from build123d import *

# Parameters (mm, degrees)
BOSS_EXTRUDE1_DEPTH             = 7.6708
SKETCH2_W                       = 5.08
SKETCH2_H                       = 0.3048
CUT_EXTRUDE1_DEPTH              = 38.1
LPATTERN1_COUNT                 = 8
LPATTERN1_PITCH                 = 0.762
F_10_32_TAPPED_HOLE1_AT_2_COUNT = 2
F_10_32_TAPPED_HOLE1_AT_2_PITCH = 19.05


with BuildPart() as part:
    # Sketch1 → Boss-Extrude1 (new body)
    with BuildSketch(Plane.XY):
        with BuildLine():
            Line((52.1716, 20.6375), (54.409054124, 20.6375))
            ThreePointArc((54.409054124, 20.6375), (54.797860491, 20.560161605), (55.127474613, 20.33992049))
            Line((55.127474613, 20.33992049), (62.03402049, 13.433374613))
            ThreePointArc((62.03402049, 13.433374613), (62.254261605, 13.103760491), (62.3316, 12.714954124))
            Line((62.3316, 12.714954124), (62.3316, 6.335045876))
            ThreePointArc((62.3316, 6.335045876), (62.254261605, 5.946239509), (62.03402049, 5.616625387))
            Line((62.03402049, 5.616625387), (60.009497552, 3.592102448))
            ThreePointArc((60.009497552, 3.592102448), (58.5216, 0), (60.009497552, -3.592102448))
            Line((60.009497552, -3.592102448), (62.03402049, -5.616625387))
            ThreePointArc((62.03402049, -5.616625387), (62.254261605, -5.946239509), (62.3316, -6.335045876))
            Line((62.3316, -6.335045876), (62.3316, -12.714954124))
            ThreePointArc((62.3316, -12.714954124), (62.254261605, -13.103760491), (62.03402049, -13.433374613))
            Line((62.03402049, -13.433374613), (55.127474613, -20.33992049))
            ThreePointArc((55.127474613, -20.33992049), (54.797860491, -20.560161605), (54.409054124, -20.6375))
            Line((54.409054124, -20.6375), (52.1716, -20.6375))
            ThreePointArc((52.1716, -20.6375), (50.914364143, -20.116735857), (50.3936, -18.8595))
            Line((50.3936, -18.8595), (50.3936, 18.8595))
            ThreePointArc((50.3936, 18.8595), (50.914364143, 20.116735857), (52.1716, 20.6375))
        make_face()
    extrude(amount=-BOSS_EXTRUDE1_DEPTH)

    # Sketch2 → Cut-Extrude1 (cut, symmetric)
    with BuildSketch(Plane(origin=(0, 0, 0), x_dir=(1, 0, 0), z_dir=(0, 1, 0))):
        with Locations((49.4284, 0.9144)):
            Rectangle(SKETCH2_W, SKETCH2_H)
    cut_extrude1 = extrude(amount=CUT_EXTRUDE1_DEPTH, both=True, mode=Mode.SUBTRACT)

    # LPattern1: Cut-Extrude1 ×8
    with Locations(*[(0, 0, -i * LPATTERN1_PITCH) for i in range(1, LPATTERN1_COUNT)]):
        add(cut_extrude1, mode=Mode.SUBTRACT)

    # Sketch3 → #10-32 Tapped Hole1 (revolve, cut)
    with BuildSketch(Plane(origin=(56.3626, 9.525, 0), x_dir=(0, -1, 0), z_dir=(1, 0, 0))):
        Polygon((0, 0), (0, 7.6708), (2.54, 7.6708), (2.0193, 7.1501), (2.0193, 0.5207), (2.54, 0), align=None)
    f_10_32_tapped_hole1 = revolve(axis=Axis((56.3626, 9.525, 6.35), (0, 0, -1)), mode=Mode.SUBTRACT)

    # #10-32 Tapped Hole1 at 2: #10-32 Tapped Hole1 ×2
    with Locations(*[(0, -i * F_10_32_TAPPED_HOLE1_AT_2_PITCH, 0) for i in range(1, F_10_32_TAPPED_HOLE1_AT_2_COUNT)]):
        add(f_10_32_tapped_hole1, mode=Mode.SUBTRACT)


solid = part.part
Work out the finished part from the listing and answer in its coordinate system (mm). A direction names the side the tool comes from. Coordinates: 2 decimals unless noted, no trailing zeros. Write each loop counter-clockwise with the first axis right and the second up, starting at its lowest first coordinate (ties: lowest second). Pieces come first, ordered by that corner, then holes.
1. For faces 4 (the flat face through (51, 0, -5.639)), 5 (the flat face through (61.04, 4.62, -3.78)), 6 (the flat face through (55, 0, 0)), determine the directions among +Z, -Z, +X, -X, +Y, -Y from which every point of the face is accessible in a straight line to the end or side of a thin tool.
Results list:
face 4: -X, +Y, -Y
face 5: +Z, -Z, +X
face 6: +Z, +X, -X, +Y, -Y
2. Consider line 1 along Y through (x, z) = (55, -1); line 2 along Y through (x, z) = (57, -6.75); line 3 along X through (y, z) = (7, -1). Determine where each line is inside the solid, lowest interval first.
Results list:
line 1: y = -20.45 to -11.02, -8.03 to 8.03, 11.02 to 20.45
line 2: y = -18.47 to -11.44, -7.61 to 7.61, 11.44 to 18.47
line 3: x = 51.97 to 62.33
3. For a pull along X with two mould halves and no side action, classify faces 1 (the flat face through (55, 0, -7.671)), 2 (the flat face through (58.63, -16.84, -3.78)), 3 (the cylindrical face through (58.154, -10.457, -3.789)) as +X half, -X half, draft (parallel to the pull), parting line (faces both ways), or undercut.
Results list:
face 1: draft
face 2: +X half
face 3: undercut
4. The part is cut by section B-B, the plane x = 51.5. State how many separate pieces and enclosed holes the cut face has, and give its area (3 significant figures).
Results list:
separate pieces: 9
enclosed holes: 0
area: 215 mm2
5. The part is cut by section A-A, the plane x = 60.75. Write down the section's boundary in (y, z).
Results list:
outline: (-14.72, -7.67) - (-4.33, -7.67) - (-4.33, 0) - (-14.72, 0) - close; (4.33, -7.67) - (14.72, -7.67) - (14.72, 0) - (4.33, 0) - close
6. A flat-ended cylindrical pin translates along its axis: pin 1 (3 mm diameter, centred on y = 0, z = -2, fed in from +X). Find the tip coordinate at first contact, or state that the pin passes through.
Results list:
pin 1: stops at x = 58.75
